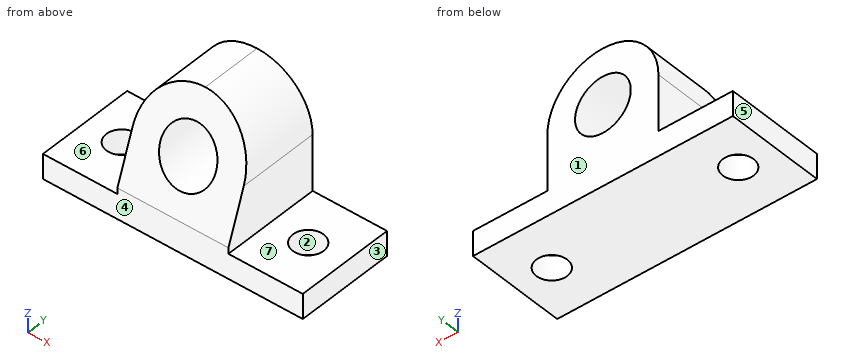
from build123d import *

# Parameters (mm, degrees)
F0_W     = 50.8
F0_H     = 12.7
F0_H_2   = 3.048
F1_DEPTH = 56.896
F2_DEPTH = 94.996
F3_DEPTH = 38.1
F4_R     = 28.44799
F6_DEPTH = 51.054
F8_DEPTH = 42.418


# Not quite as in the source:
# - a fillet or chamfer is up to 0.001 mm smaller than in the source, because OpenCascade refuses the exact size


with BuildPart() as f1:
    # F0 (on Right) → F1 (new body)
    with BuildSketch(Plane.YZ):
        with Locations((25.4, 6.35)):
            Rectangle(F0_W, F0_H)
        Polygon((19.5990691748, 69.596), (0, 15.748), (50.8, 15.748), (50.8, 69.596), align=None)
        with Locations((25.4, 14.224)):
            Rectangle(F0_W, F0_H_2)
    extrude(amount=F1_DEPTH)

    # F0 (on Right) → F2 (join)
    with BuildSketch(Plane.YZ):
        with Locations((25.4, 6.35)):
            Rectangle(F0_W, F0_H)
    extrude(amount=F2_DEPTH)

    # F0 (on Right) → F3 (join)
    with BuildSketch(Plane.YZ):
        with Locations((25.4, 6.35)):
            Rectangle(F0_W, F0_H)
    extrude(amount=-F3_DEPTH)

    # F4 (radius 28.448 in the source; OpenCascade refuses exactly that, so slightly less here)
    f4_edges = [f1.edges().sort_by_distance(p)[0] for p in [
        (0, 35.199535, 69.596),
        (56.896, 35.199535, 69.596),
    ]]
    fillet(f4_edges, radius=F4_R)

    # F5 (on face) → F6 (cut)
    with BuildSketch(Plane(origin=(0, 50.8, 0), x_dir=(-1, 0, 0), z_dir=(0, 1, 0))):
        with BuildLine():
            ThreePointArc((-14.1605, 41.148), (-28.448, 55.4355), (-42.7355, 41.148))
            Line((-42.7355, 41.148), (-14.1605, 41.148))
        make_face()
        with BuildLine():
            Line((-14.1605, 41.148), (-42.7355, 41.148))
            ThreePointArc((-42.7355, 41.148), (-28.448, 26.8605), (-14.1605, 41.148))
        make_face()
    extrude(amount=-F6_DEPTH, mode=Mode.SUBTRACT)

    # F7 (on face) → F8 (cut)
    with BuildSketch(Plane(origin=(0, 0, 0), x_dir=(1, 0, 0), z_dir=(0, 0, -1))):
        with BuildLine():
            ThreePointArc((-11.43, -25.4), (-19.304, -17.526), (-27.178, -25.4))
            Line((-27.178, -25.4), (-19.304, -25.4))
            Line((-19.304, -25.4), (-11.43, -25.4))
        make_face()
        with BuildLine():
            ThreePointArc((84.074, -25.4), (76.2, -17.526), (68.326, -25.4))
            Line((68.326, -25.4), (76.2, -25.4))
            Line((76.2, -25.4), (84.074, -25.4))
        make_face()
        with BuildLine():
            Line((76.2, -25.4), (68.326, -25.4))
            ThreePointArc((68.326, -25.4), (76.2, -33.274), (84.074, -25.4))
            Line((84.074, -25.4), (76.2, -25.4))
        make_face()
        with BuildLine():
            Line((-19.304, -25.4), (-27.178, -25.4))
            ThreePointArc((-27.178, -25.4), (-19.304, -33.274), (-11.43, -25.4))
            Line((-11.43, -25.4), (-19.304, -25.4))
        make_face()
    extrude(amount=-F8_DEPTH, mode=Mode.SUBTRACT)


solid = f1.part
For this review, take the finished solid that the model builds, in its own axes (mm). Face numbers are marked on the shaded views. A direction names the side the tool comes from. Round coordinates to 2 decimals unless told otherwise and drop trailing zeros. Write each loop counter-clockwise with the first axis right and the second up, starting at its lowest first coordinate (ties: lowest second). Pieces come first, ordered by that corner, then holes. Notation, with made-up numbers: (-5.5, 80.25) -> (25.5, 80.25) arc R15 ccw to (25.5, 101.25) -> close; hole circle Ø2 at (75.25, 4.25). An arc over 180 degrees is marked (long way). Put each result on its own line as item: value.
Q1. Consider section C-C on z = 50.5. State the section outline as (x, y) points.
Determined:
outline: (1.58, 12.65) -> (17.65, 12.65) -> (17.65, 50.8) -> (1.58, 50.8) -> close; (39.25, 12.65) -> (55.31, 12.65) -> (55.31, 50.8) -> (39.25, 50.8) -> close
Q2. The part is to be moulded in two halves that separate along Y. For the marked faces 1, 2, 3 and 4, say which applies: released by +Y, released by -Y, zero draft, split by the parting line, or undercut.
Determined:
face 1: released by +Y
face 2: undercut
face 3: zero draft
face 4: released by -Y
Q3. Machinability: for the marked faces 5, 6 and 7, which of the approach directions +Z, -Z, +X, -X, +Y, -Y give a long, thin tool a straight path to every point of the face, cutting with its end or side? Answer none if there is none.
Determined:
face 5: +Z, -Z, -X, +Y, -Y
face 6: +Z, -X, +Y, -Y
face 7: +Z, +X, +Y, -Y
Q4. Consider section A-A on y = 25.4. Give the number of separate pieces and of enclosed holes in the cut face, and give its area (3 significant figures).
Determined:
separate pieces: 3
enclosed holes: 1
area: 3,540 mm^2
Q5. To check wall thickness, follow L1, parallel to X at y = 25, z = 6; L2, parallel to Y at x = 76.2, z = 9.75; L3, parallel to X at y = 11.5, z = 41.5. State the ranges of each line that lie inside material, in increasing order. Write a range as [from, to].
Determined:
L1: x = [-38.1, -27.17], [-11.44, 68.34], [84.06, 95]
L2: y = [0, 17.53], [33.27, 50.8]
L3: x = [0, 14.16], [42.73, 56.89]
Q6. Clearance check with flat-ended pins moving along their axes: pin 1 Ø19 at (x, y) = (79, 26.5) entering from +Z; pin 2 Ø12 at (y, z) = (18, 28.5) entering from -X; pin 3 Ø14 at (y, z) = (35.5, 23.5) entering from +X. State where each tip first meets the part, or that it passes through.
Determined:
pin 1: stops at z = 12.7
pin 2: stops at x = 0
pin 3: stops at x = 56.9
Q7. Consider section B-B on x = 76.2. State the section outline as (y, z) points.
Determined:
outline: (0, 0) -> (17.53, 0) -> (17.53, 12.7) -> (0, 12.7) -> close; (33.27, 0) -> (50.8, 0) -> (50.8, 12.7) -> (33.27, 12.7) -> close
Q8. Consider section D-D on y = 12. State the section outline as (x, z) points (1 decimal).
Determined:
outline: (-38.1, 0) -> (95, 0) -> (95, 12.7) -> (56.9, 12.7) -> (56.9, 41.1) arc R28.4 ccw to (55.9, 48.7) -> (40.6, 48.7) arc R14.3 cw (long way) to (16.3, 48.7) -> (1, 48.7) arc R28.4 ccw to (0, 41.1) -> (0, 12.7) -> (-38.1, 12.7) -> close
